```python
from build123d import *

# Parameters (mm, degrees)
F3_R      = 0.15
F4_DEPTH  = 4
F3_R_2    = 0.85
F6_DEPTH  = 1
F8_DEPTH  = 2.25
F10_DEPTH = 0.75
F14_W     = 1.02
F14_H     = 2.5
F15_DEPTH = 0.2


with BuildPart() as f4:
    # F3 (on Top) → F4 (new body)
    with BuildSketch(Plane.XY):
        with Locations((-3.35, -1)):
            Circle(F3_R)
    extrude(amount=F4_DEPTH)


with BuildPart() as f4b:
    # F3 (on Top) → F4, piece 2 (new body)
    with BuildSketch(Plane.XY):
        with BuildLine():
            ThreePointArc((-0.6479896557, 1.7900277778), (-0.6125199075, 1.8400064655), (-0.6, 1.9))
            ThreePointArc((-0.6, 1.9), (-0.8099935345, 2.0374800925), (-0.8520103443, 1.7900277778))
            ThreePointArc((-0.8520103443, 1.7900277778), (-0.75, 1.805), (-0.6479896557, 1.7900277778))
        make_face()
        with BuildLine():
            ThreePointArc((-0.6479896557, 1.7900277778), (-0.75, 1.805), (-0.8520103443, 1.7900277778))
            ThreePointArc((-0.8520103443, 1.7900277778), (-0.75, 1.75), (-0.6479896557, 1.7900277778))
        make_face()
        with BuildLine():
            ThreePointArc((-0.6479896557, 1.7900277778), (-0.75, 1.75), (-0.8520103443, 1.7900277778))
            ThreePointArc((-0.8520103443, 1.7900277778), (-0.9619095654, 1.1651854356), (-0.395, 1.45))
            ThreePointArc((-0.395, 1.45), (-0.4651854356, 1.6619095654), (-0.6479896557, 1.7900277778))
        make_face()
    extrude(amount=F4_DEPTH)


with BuildPart() as f4c:
    # F3 (on Top) → F4, piece 3 (new body)
    with BuildSketch(Plane.XY):
        with Locations((-0.35, 2.4)):
            Circle(F3_R)
    extrude(amount=F4_DEPTH)


with BuildPart() as f4d:
    # F3 (on Top) → F4, piece 4 (new body)
    with BuildSketch(Plane.XY):
        with Locations((2.5, -2.6)):
            Circle(F3_R_2)
    extrude(amount=F4_DEPTH)


with BuildPart() as f6:
    # F5 (on face) → F6 (new body)
    with BuildSketch(Plane.XY.offset(4)):
        with BuildLine():
            ThreePointArc((1.9858394431, -1.8458978499), (2.7430307581, -0.5560249217), (2.2269639391, 0.8478218992))
            Line((2.2269639391, 0.8478218992), (0.1407855756, 2.8991287597))
            ThreePointArc((0.1407855756, 2.8991287597), (-0.3747911939, 3.0995608599), (-0.8748864988, 2.863135146))
            Line((-0.8748864988, 2.863135146), (-3.8748864988, -0.536864854))
            ThreePointArc((-3.8748864988, -0.536864854), (-3.9698749845, -0.674800056), (-4.0293801406, -0.831350587))
            Line((-4.0293801406, -0.831350587), (-4.695, -3.5127053911))
            Line((-4.695, -3.5127053911), (-4.695, -4.5127053911))
            Line((-4.695, -4.5127053911), (4.695, -4.5127053911))
            Line((4.695, -4.5127053911), (4.695, -4.0127053911))
            ThreePointArc((4.695, -4.0127053911), (4.5485533906, -3.6591520005), (4.195, -3.5127053911))
            Line((4.195, -3.5127053911), (2.5, -3.5127053911))
            ThreePointArc((2.5, -3.5127053911), (1.6278462782, -2.869033486), (1.9858394431, -1.8458978499))
        make_face()
    extrude(amount=-F6_DEPTH)

    # F7 (on face) → F8 (join)
    with BuildSketch(Plane(origin=(0, 0, 3), x_dir=(1, 0, 0), z_dir=(0, 0, -1))):
        with BuildLine():
            ThreePointArc((0.645, 3.8677053911), (0.2746634171, 4.4513020046), (-0.411077542, 4.3647368333))
            Line((-0.411077542, 4.3647368333), (-3.429889044, 1.8679820876))
            ThreePointArc((-3.429889044, 1.8679820876), (-3.6098399318, 1.5198675017), (-3.4835090032, 1.1489138881))
            Line((-3.4835090032, 1.1489138881), (-0.75, -1.9))
            Line((-0.75, -1.9), (-0.35, -2.4))
            Line((-0.35, -2.4), (1.7282178972, -0.3565205426))
            ThreePointArc((1.7282178972, -0.3565205426), (1.840398747, 0.1893934116), (1.3776567718, 0.5))
            Line((1.3776567718, 0.5), (1.3406244266, 0.5))
            ThreePointArc((1.3406244266, 0.5), (1.0505140008, 0.0486122715), (0.645, 0.4))
            Line((0.645, 0.4), (0.645, 3.8677053911))
        make_face()
    extrude(amount=F8_DEPTH)

    # F9 (on face) → F10 (join)
    with BuildSketch(Plane(origin=(0, 0, 0.75), x_dir=(1, 0, 0), z_dir=(0, 0, -1))):
        with BuildLine():
            ThreePointArc((-3.7485538053, 2.2532777792), (-4.1598651003, 1.4614479318), (-3.8772413796, 0.6151056127))
            Line((-3.8772413796, 0.6151056127), (-0.837394606, -2.8300540641))
            ThreePointArc((-0.837394606, -2.8300540641), (-0.3730203944, -3.049592227), (0.1057294631, -2.8634767054))
            Line((0.1057294631, -2.8634767054), (2.1839473603, -0.8199972481))
            ThreePointArc((2.1839473603, -0.8199972481), (2.5083795632, 0.2096806356), (1.8363283859, 1.054571169))
            ThreePointArc((1.8363283859, 1.054571169), (1.3332379826, 1.4786553659), (1.145, 2.1091423379))
            Line((1.145, 2.1091423379), (1.145, 3.8677053911))
            ThreePointArc((1.145, 3.8677053911), (0.4875807948, 4.9037024802), (-0.7297423032, 4.7500325249))
            Line((-0.7297423032, 4.7500325249), (-3.7485538053, 2.2532777792))
        make_face()
    extrude(amount=F10_DEPTH)

    # F11: cut F4, F4b, F4c, F4d
    add(f4.part, mode=Mode.SUBTRACT)
    add(f4b.part, mode=Mode.SUBTRACT)
    add(f4c.part, mode=Mode.SUBTRACT)
    add(f4d.part, mode=Mode.SUBTRACT)

    # F13: sweep along a path in F12
    with BuildLine(Plane.YZ) as f13_path:
        Line((-9.0232299709, 5.641696688), (-4.5127053911, 4))
    # F6_face1 (on face) → F13 (sweep)
    with BuildSketch(Plane(origin=(0, -4.5127053911, 3.5), x_dir=(1, 0, 0), z_dir=(0, -1, 0))):
        Polygon((-4.695, 0.5), (-4.695, -0.5), (0, -0.5), (4.695, -0.5), (4.695, 0.5), align=None)
    sweep(path=f13_path.line)

    # F14 (on face) → F15 (cut)
    with BuildSketch(Plane(origin=(0, 0.757688968, 2.0817333304), x_dir=(1, 0, 0), z_dir=(0, 0.3420201433, 0.9396926208))):
        with Locations((-3.81, -9.1586365291)):
            Rectangle(F14_W, F14_H)
        with Locations((-2.54, -9.1586365291)):
            Rectangle(F14_W, F14_H)
        with Locations((-1.27, -9.1586365291)):
            Rectangle(F14_W, F14_H)
        with Locations((0, -9.1586365291)):
            Rectangle(F14_W, F14_H)
        with Locations((1.27, -9.1586365291)):
            Rectangle(F14_W, F14_H)
        with Locations((2.54, -9.1586365291)):
            Rectangle(F14_W, F14_H)
        with Locations((3.81, -9.1586365291)):
            Rectangle(F14_W, F14_H)
    extrude(amount=-F15_DEPTH, mode=Mode.SUBTRACT)


solid = f6.part
```
Check sheet for the modelled part. Datum: model origin and axes. Units: mm. A direction names the side the tool comes from. Round coordinates to 2 decimals unless told otherwise and drop trailing zeros. Write each loop counter-clockwise with the first axis right and the second up, starting at its lowest first coordinate (ties: lowest second). Pieces come first, ordered by that corner, then holes. Notation, with made-up numbers: M 17,9.5 L 67,9.5 A20 cw 67,27.5 Z; hole C 21.25,24.25 d1. An arc over 180 degrees is marked long. Write item = value, one per line. Start each with the question number.
1. Tool access check on faces 1 (the flat face through (2.53, -7.87, 5.01)), 2 (the flat face through (-1, -1, 4)), 3 (the flat face through (1, -1, 0.75)), 4 (the flat face through (-4.358, -2.153, 3.507)). Record the directions out of +Z, -Z, +X, -X, +Y, -Y that give a thin tool (end or side, any length) a straight path to the whole face; none if there is none.
2. Scan lines: line 1 (Z direction, x = 2.25, y = -0.5); line 2 (X direction, y = 2.5, z = 0.7); line 3 (X direction, y = -1, z = 2.15) (3 decimals). Record each from-to range of solid material in increasing order. Write a range as [from, to].
3. Section check D-D, the plane x = 1. Record the cut outline in (y, z) (3 decimals).
4. Release check for a two-part mould opening along Z. For faces 5 (the flat face through (3.4, -3.513, 3.5)), 6 (the flat face through (0.07, -6.24, 4.63)), 7 (the cylindrical face through (1.843, -0.182, 1.891)), 8 (the flat face through (-2.19, 0.294, 1.891)) record: pulls with the +Z half, pulls with the -Z half, needs draft (parallel to the pull), parting line crosses it, or undercut.
5. Section check A-A, the plane x = 3.75. Record the cut outline in (y, z).
6. Gauge pin test, flat ends, axial feed: pin 1 (3 mm diameter, centred on x = -1, y = -0.5, fed in from -Z); pin 2 (5.5 mm diameter, centred on x = -2, y = -2.5, fed in from +Z); pin 3 (4 mm diameter, centred on x = -1, y = 0, fed in from +Z); pin 4 (3 mm diameter, centred on x = 0, z = 1.5, fed in from -Y). Record the tip position at first contact, or that the pin passes through.
7. Section check C-C, the plane y = -5.75. Record the cut outline in (x, z) (3 decimals), then the cut area to 3 significant figures.
Results found:
q1.face_1 = +Z
q1.face_2 = +Z, +X, -X, +Y
q1.face_3 = none
q1.face_4 = +Z, -X, +Y
q2.line_1 = [0, 0.75], [3, 4]
q2.line_2 = [-1.13, -0.46], [-0.24, 0.48]
q2.line_3 = [-3.2, 0.645]
q3.outline = M -9.023,4.642 L -4.513,3 L -0.045,3 L -0.045,0.75 L -4.425,0.75 L -4.425,0 L 1.984,0 L 1.984,0.75 L 1.073,0.75 L 1.073,3 L 2.054,3 L 2.054,4 L -4.513,4 L -6.674,4.787 L -6.742,4.599 L -9.023,5.429 Z
q4.face_5 = needs draft
q4.face_6 = pulls with the +Z half
q4.face_7 = undercut
q4.face_8 = undercut
q5.outline = M -9.02,4.64 L -4.51,3 L -3.51,3 L -3.51,4 L -4.51,4 L -6.67,4.79 L -6.74,4.6 L -9.02,5.43 Z
q6.pin_1 = 0
q6.pin_2 = 4.27
q6.pin_3 = 4
q6.pin_4 = -5.01
q7.outline = M -4.695,3.45 L 4.695,3.45 L 4.695,4.45 L -4.695,4.45 Z
q7.area = 9.39 mm^2
